from build123d import *

# Parameters (mm, degrees)
F1_DEPTH = 50
F3_D     = 4
F3_DEPTH = 10
F2_W     = 8
F2_H     = 26
F4_DEPTH = 25


with BuildPart() as f1:
    # F0 (on Top) → F1 (new body)
    with BuildSketch(Plane.XY):
        with BuildLine():
            Line((0, 0), (15, 0))
            Line((15, 0), (15, 1))
            Line((15, 1), (0, 1))
            ThreePointArc((0, 1), (-1.414214, 4.414214), (2, 3))
            Line((2, 3), (2, 2))
            Line((2, 2), (3, 2))
            Line((3, 2), (3, 3))
            ThreePointArc((3, 3), (-2.12132, 5.12132), (0, 0))
        make_face()
    extrude(amount=F1_DEPTH)

    # F3
    with Locations(Plane.XZ):
        with Locations((10, 45), (7, 25), (10, 5)):
            Hole(F3_D / 2, depth=F3_DEPTH)

    # F2 (on Front) → F4 (cut)
    with BuildSketch(Plane.XZ):
        with Locations((-1, 25)):
            Rectangle(F2_W, F2_H)
    extrude(amount=-F4_DEPTH, mode=Mode.SUBTRACT)


solid = f1.part
Model file for the job. Use its own axes, mm. A direction names the side the tool comes from. Give positions to 0.01 mm unless a question says otherwise; leave off trailing zeros. Order: outer loops, then holes, each group sorted by start corner. A loop starts at its lowest first (then second) coordinate and runs counter-clockwise, first axis right, second up. Notation, with made-up numbers: (79.25, -13) - (131.25, -13) arc R15 cw to (131.25, -2) - close; hole circle Ø11 at (-11.5, -5). An arc over 180 degrees is marked (long way). Write item = value, one per line. Start each with the question number.
1. Two-plate mould, pull along Z, no slides. Class faces 5 (the flat face through (9.3, 1, 24.6)), 6 (the flat face through (2.6, 2.6, 0)), 7 (the cylindrical face through (8.6, 0.5, 23.8)): pulls with the +Z half, pulls with the -Z half, needs draft (parallel to the pull), parting line crosses it, or undercut.
2. Cut at B-B, the plane x = 7. List the corners of the cut face in (y, z), and give its area (3 significant figures).
3. Which spindle directions (+Z, -Z, +X, -X, +Y, -Y) get a long thin tool onto all of the face, cutting with end or side? Do faces 1 (the flat face through (2.5, 2, 43.9)), 2 (the flat face through (3, 0.5, 24.8)), 3 (the flat face through (2, 2.5, 5.9)), 4 (the flat face through (3, 2.5, 5.9)). Say none if no direction does.
4. Drop flat-ended pins along their axis: P1, Ø0.8, axis at y = 2.5, z = 44, coming from the +X side; P2, Ø6.5, axis at x = 10, z = 5, coming from the +Y side; P3, Ø2.5, axis at x = 0, y = 3, coming from the +Z side; P4, Ø0.5, axis at y = 0.5, z = 24.5, coming from the -X side. Give the stop position or say it passes through.
5. Cut at D-D, the plane z = 9. List the corners of the cut face in (x, y), and give its area (3 significant figures).
6. Cut at A-A, the plane z = 25. List the corners of the cut face in (x, y), and give its area (3 significant figures).
7. Cut at C-C, the plane y = 3.6. List the corners of the cut face in (x, z), and give its area (3 significant figures).
8. Probe line 1 along Z through (x, y) = (10, 0.5); line 2 along Y through (x, z) = (0, 3); line 3 along Z through (x, y) = (7, 0.65). List the from-to ranges inside material, lowest first.
Taken from the geometry:
q1.face_5 = needs draft
q1.face_6 = pulls with the -Z half
q1.face_7 = undercut
q2.outline = (0, 0) - (1, 0) - (1, 23) - (0, 23) - close; (0, 27) - (1, 27) - (1, 50) - (0, 50) - close
q2.area = 46.0 mm²
q3.face_1 = +Z, -Z, +X
q3.face_2 = -X, +Y, -Y
q3.face_3 = +Z, -Z
q3.face_4 = +Z, -Z, +X, +Y
q4.P1 = 3
q4.P2 = 1
q4.P3 = through
q4.P4 = 3
q5.outline = (0, 0) - (15, 0) - (15, 1) - (0, 1) arc R2 cw (long way) to (2, 3) - (2, 2) - (3, 2) - (3, 3) arc R3 ccw (long way) to start
q5.area = 27.8 mm²
q6.outline = (3, 0) - (5, 0) - (5, 1) - (3, 1) - close; (9, 0) - (15, 0) - (15, 1) - (9, 1) - close
q6.area = 8.00 mm²
q7.outline = (-2.94, 0) - (-1.91, 0) - (-1.91, 12) - (-2.94, 12) - close; (-2.94, 38) - (-1.91, 38) - (-1.91, 50) - (-2.94, 50) - close; (1.91, 0) - (2.94, 0) - (2.94, 12) - (1.91, 12) - close; (1.91, 38) - (2.94, 38) - (2.94, 50) - (1.91, 50) - close
q7.area = 49.5 mm²
q8.line_1 = 0 to 3, 7 to 43, 47 to 50
q8.line_2 = 0 to 1, 5 to 6
q8.line_3 = 0 to 23, 27 to 50
